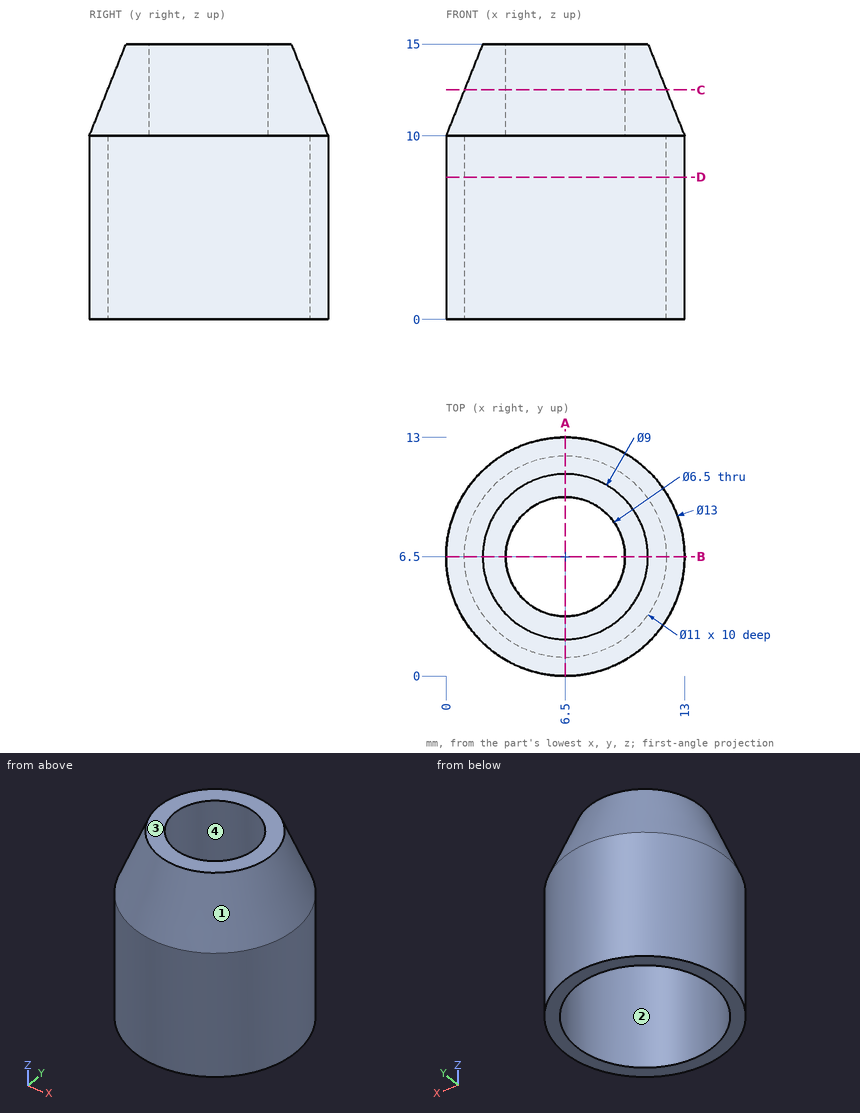
Geometry check sheet. Reference: drawing and pictorial views, mm from the part's lowest x, y, z. Round coordinates to 2 decimals unless told otherwise and drop trailing zeros. Write each loop counter-clockwise with the first axis right and the second up, starting at its lowest first coordinate (ties: lowest second). Pieces come first, ordered by that corner, then holes.
1. Gauge pin test, flat ends, axial feed: P1, Ø1.5, axis at y = 10, z = 6, coming from the +X side; P2, Ø3, axis at x = 3.5, z = 2, coming from the -Y side; P3, Ø4, axis at y = 10, z = 11, coming from the -X side. Record the tip position at first contact, or that the pin passes through.
2. Scan lines: L1, parallel to X at y = 6.5, z = 2.75; L2, parallel to Z at x = 6, y = 2.75. Record each from-to range of solid material in increasing order.
3. Section check A-A on x = 6.5. Enter the section's corners in (y, z), plus the area to 3 significant figures.
4. Section check C-C on z = 12.5. Enter the section's corners in (x, y), plus the area to 4 significant figures.
5. Section check D-D on z = 7.75. Enter the section's corners in (x, y).
6. Draft check along X on the marked faces 1, 2, 3 and 4. Enter one of: +X half, -X half, draft (parallel to the pull), parting line (faces both ways), or undercut.
Answer:
1. P1: stops at x = 12.39
1. P2: stops at y = 0.18
1. P3: stops at x = 0.25
2. L1: x = 0 to 1, 12 to 13
2. L2: z = 10 to 15
3. outline: (0, 0) - (1, 0) - (1, 10) - (3.25, 10) - (3.25, 15) - (2, 15) - (0, 10) - close; (9.75, 10) - (12, 10) - (12, 0) - (13, 0) - (13, 10) - (11, 15) - (9.75, 15) - close
3. area: 42.5 mm2
4. outline: circle Ø11 at (6.5, 6.5); hole circle Ø6.5 at (6.5, 6.5)
4. area: 61.85 mm2
5. outline: circle Ø13 at (6.5, 6.5); hole circle Ø11 at (6.5, 6.5)
6. face 1: parting line
6. face 2: undercut
6. face 3: draft
6. face 4: undercut
